from build123d import *

# Parameters (mm, degrees)
SKETCH1_W           = 203.2
SKETCH1_H           = 127
BOSS_EXTRUDE1_DEPTH = 3.175
SKETCH3_W           = 40.64
SKETCH3_H           = 3.175
CUT_EXTRUDE1_DEPTH  = 3.175
LPATTERN1_COUNT     = 2
LPATTERN1_PITCH     = 81.28
SKETCH5_W           = 40.64
SKETCH5_H           = 3.175
CUT_EXTRUDE2_DEPTH  = 3.175
LPATTERN2_COUNT     = 2
LPATTERN2_PITCH     = 81.28
SKETCH6_W           = 3.175
SKETCH6_H           = 25.4
CUT_EXTRUDE3_DEPTH  = 3.175
LPATTERN3_COUNT     = 2
LPATTERN3_PITCH     = 50.8
SKETCH7_W           = 3.175
SKETCH7_H           = 25.4
CUT_EXTRUDE4_DEPTH  = 3.175
LPATTERN4_COUNT     = 2
LPATTERN4_PITCH     = 50.8


with BuildPart() as part:
    # Sketch1 → Boss-Extrude1 (new body)
    with BuildSketch(Plane(origin=(0, 0, 0), x_dir=(1, 0, 0), z_dir=(0, 1, 0))):
        Rectangle(SKETCH1_W, SKETCH1_H)
    extrude(amount=BOSS_EXTRUDE1_DEPTH)

    # Sketch3 → Cut-Extrude1 (cut)
    with BuildSketch(Plane(origin=(0, 3.175, 0), x_dir=(1, 0, 0), z_dir=(0, 1, 0))):
        with Locations((-40.64, -61.9125)):
            Rectangle(SKETCH3_W, SKETCH3_H)
    cut_extrude1 = extrude(amount=-CUT_EXTRUDE1_DEPTH, mode=Mode.SUBTRACT)

    # LPattern1: Cut-Extrude1 ×2
    with Locations(*[(i * LPATTERN1_PITCH, 0, 0) for i in range(1, LPATTERN1_COUNT)]):
        add(cut_extrude1, mode=Mode.SUBTRACT)

    # Sketch5 → Cut-Extrude2 (cut)
    with BuildSketch(Plane(origin=(0, 3.175, 0), x_dir=(1, 0, 0), z_dir=(0, 1, 0))):
        with Locations((-40.64, 61.9125)):
            Rectangle(SKETCH5_W, SKETCH5_H)
    cut_extrude2 = extrude(amount=-CUT_EXTRUDE2_DEPTH, mode=Mode.SUBTRACT)

    # LPattern2: Cut-Extrude2 ×2
    with Locations(*[(i * LPATTERN2_PITCH, 0, 0) for i in range(1, LPATTERN2_COUNT)]):
        add(cut_extrude2, mode=Mode.SUBTRACT)

    # Sketch6 → Cut-Extrude3 (cut)
    with BuildSketch(Plane(origin=(0, 3.175, 0), x_dir=(1, 0, 0), z_dir=(0, 1, 0))):
        with Locations((-100.0125, -25.4)):
            Rectangle(SKETCH6_W, SKETCH6_H)
    cut_extrude3 = extrude(amount=-CUT_EXTRUDE3_DEPTH, mode=Mode.SUBTRACT)

    # LPattern3: Cut-Extrude3 ×2
    with Locations(*[(0, 0, -i * LPATTERN3_PITCH) for i in range(1, LPATTERN3_COUNT)]):
        add(cut_extrude3, mode=Mode.SUBTRACT)

    # Sketch7 → Cut-Extrude4 (cut)
    with BuildSketch(Plane(origin=(0, 3.175, 0), x_dir=(1, 0, 0), z_dir=(0, 1, 0))):
        with Locations((100.0125, -25.4)):
            Rectangle(SKETCH7_W, SKETCH7_H)
    cut_extrude4 = extrude(amount=-CUT_EXTRUDE4_DEPTH, mode=Mode.SUBTRACT)

    # LPattern4: Cut-Extrude4 ×2
    with Locations(*[(0, 0, -i * LPATTERN4_PITCH) for i in range(1, LPATTERN4_COUNT)]):
        add(cut_extrude4, mode=Mode.SUBTRACT)


solid = part.part
Input: part model. Units: mm. Frame: model coordinates. Coordinates: 2 decimals unless noted, no trailing zeros. Loops run counter-clockwise (first coordinate to the right, second up) from the corner with the lowest first, then second, coordinate; pieces in that order, holes last. Notation, with made-up numbers: (-9.5, -27.5) - (6.5, -27.5) arc R24 cw to (6.5, 11.5) - close; hole circle Ø10 at (1.5, 15.5). An arc over 180 degrees is marked (long way). Answer in a Markdown table with one row per item. Add a question column.
Item 1: Section query A-A on x = -46.5. Return the cut outline in (y, z) (3 decimals).
Item 2: Line query: line 1 along X through (y, z) = (0.2, 28) (3 decimals); line 2 along Z through (x, y) = (29.5, 0.6) (3 decimals). Output: solid intervals per line, ascending. Write a range as [from, to].
Item 3: Section query B-B on z = -25. Return the cut outline in (x, y) (3 decimals), then the cut area to 3 significant figures.
Item 4: Contact query for flat-ended pins moving along their axis: P1, Ø1.6, axis at x = -44, y = 1, coming from the +Z side (3 decimals); P2, Ø1.6, axis at x = -36.5, y = 2, coming from the -Z side (3 decimals); P3, Ø1, axis at y = 2, z = -22, coming from the +X side (3 decimals). Output: stop coordinate, or through.
Recorded:
| question | item | result |
|---|---|---|
| 1 | outline | (0, -60.325) - (3.175, -60.325) - (3.175, 60.325) - (0, 60.325) - close |
| 2 | line 1 | [-98.425, 98.425] |
| 2 | line 2 | [-60.325, 60.325] |
| 3 | outline | (-98.425, 0) - (98.425, 0) - (98.425, 3.175) - (-98.425, 3.175) - close |
| 3 | area | 625 mm^2 |
| 4 | P1 | z = 60.325 |
| 4 | P2 | z = -60.325 |
| 4 | P3 | x = 98.425 |
